For this review, take the finished solid that the model builds, in its own axes (mm). Face numbers are marked on the shaded views. A direction names the side the tool comes from. Round coordinates to 2 decimals unless told otherwise and drop trailing zeros. Order: outer loops, then holes, each group sorted by start corner. A loop starts at its lowest first (then second) coordinate and runs counter-clockwise, first axis right, second up. Notation, with made-up numbers: M 60,-21 L 92,-21 A22 ccw 92,3 Z; hole C -24,-18 d4. An arc over 180 degrees is marked long. Answer as a JSON object with one key per item and string values.
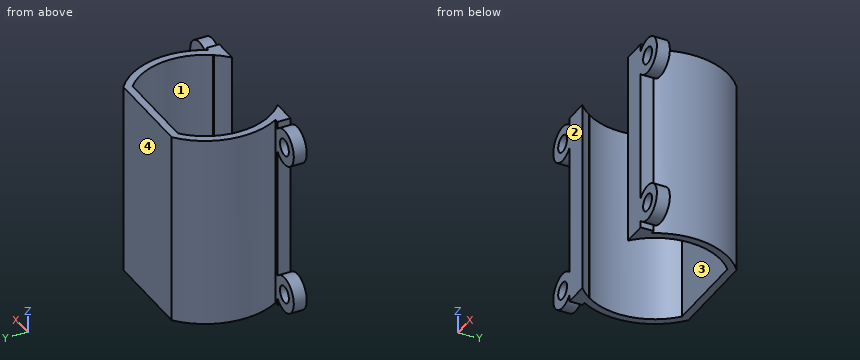
from build123d import *

# Parameters (mm, degrees)
SALIENTE_EXTRUIR1_DEPTH   = 30
VACIADO1_T                = 1.2
CROQUIS2_W                = 41.64599518
CROQUIS2_H                = 31.401201606
CORTAR_EXTRUIR1_DEPTH     = 1.3
CROQUIS3_W                = 19.002401527
CROQUIS3_H                = 2.972205444
CORTAR_EXTRUIR2_DEPTH     = 48.3
CROQUIS4_R                = 2.75
CROQUIS4_R_2              = 1.3
SALIENTE_EXTRUIR2_DEPTH   = 2
SALIENTE_EXTRUIR2_2_DEPTH = 2
SALIENTE_EXTRUIR2_3_DEPTH = 2
SALIENTE_EXTRUIR2_4_DEPTH = 2
CROQUIS5_W                = 2.061100057
CROQUIS5_H                = 29.9
SALIENTE_EXTRUIR3_DEPTH   = 2


with BuildPart() as part:
    # Croquis1 → Saliente-Extruir1 (new body)
    with BuildSketch(Plane.XY):
        with BuildLine():
            Line((-6.68954408, 7.7), (6.68954408, 7.7))
            ThreePointArc((6.68954408, 7.7), (10.2, 0), (6.68954408, -7.7))
            Line((6.68954408, -7.7), (-6.68954408, -7.7))
            ThreePointArc((-6.68954408, -7.7), (-10.2, 0), (-6.68954408, 7.7))
        make_face()
    extrude(amount=SALIENTE_EXTRUIR1_DEPTH)

    # Vaciado1
    vaciado1_openings = [part.faces().sort_by_distance(p)[0] for p in [
        (0, 0, 30),
    ]]
    offset(amount=VACIADO1_T, openings=vaciado1_openings, kind=Kind.INTERSECTION)

    # Croquis2 → Cortar-Extruir1 (cut)
    with BuildSketch(Plane(origin=(0, 0, -1.2), x_dir=(-1, 0, 0), z_dir=(0, 0, -1))):
        Rectangle(CROQUIS2_W, CROQUIS2_H)
    extrude(amount=-CORTAR_EXTRUIR1_DEPTH, mode=Mode.SUBTRACT)

    # Croquis3 → Cortar-Extruir2 (cut)
    with BuildSketch(Plane.XY.offset(30)):
        with Locations((-0.191367802, -9.186102722)):
            Rectangle(CROQUIS3_W, CROQUIS3_H)
    extrude(amount=-CORTAR_EXTRUIR2_DEPTH, mode=Mode.SUBTRACT)



with BuildPart() as body_2:
    # Croquis4 → Saliente-Extruir2 (new body)
    with BuildSketch(Plane.XZ.offset(7.7)):
        with Locations(Location((12.5, 3, 0), (0, 0, 270))):
            Circle(CROQUIS4_R)
        with Locations(Location((12.5, 3, 0), (0, 0, 270))):
            Circle(CROQUIS4_R_2, mode=Mode.SUBTRACT)
    extrude(amount=-SALIENTE_EXTRUIR2_DEPTH)


with BuildPart() as body_3:
    # Croquis4 → Saliente-Extruir2 2 (new body)
    with BuildSketch(Plane.XZ.offset(7.7)):
        with Locations(Location((12.5, 27, 0), (0, 0, 90))):
            Circle(CROQUIS4_R)
        with Locations(Location((12.5, 27, 0), (0, 0, 90))):
            Circle(CROQUIS4_R_2, mode=Mode.SUBTRACT)
    extrude(amount=-SALIENTE_EXTRUIR2_2_DEPTH)


with BuildPart() as body_4:
    # Croquis4 → Saliente-Extruir2 3 (new body)
    with BuildSketch(Plane.XZ.offset(7.7)):
        with Locations(Location((-12.5, 27, 0), (0, 0, 270))):
            Circle(CROQUIS4_R)
        with Locations(Location((-12.5, 27, 0), (0, 0, 270))):
            Circle(CROQUIS4_R_2, mode=Mode.SUBTRACT)
    extrude(amount=-SALIENTE_EXTRUIR2_3_DEPTH)


with BuildPart() as body_5:
    # Croquis4 → Saliente-Extruir2 4 (new body)
    with BuildSketch(Plane.XZ.offset(7.7)):
        with Locations(Location((-12.5, 3, 0), (0, 0, 90))):
            Circle(CROQUIS4_R)
        with Locations(Location((-12.5, 3, 0), (0, 0, 90))):
            Circle(CROQUIS4_R_2, mode=Mode.SUBTRACT)
    extrude(amount=-SALIENTE_EXTRUIR2_4_DEPTH)


with BuildPart() as part_1:
    add(part.part)

    add(body_2.part)  # Saliente-Extruir3 merges body 2

    add(body_3.part)  # Saliente-Extruir3 merges body 3

    add(body_4.part)  # Saliente-Extruir3 merges body 4

    add(body_5.part)  # Saliente-Extruir3 merges body 5
    # Croquis5 → Saliente-Extruir3 (add)
    with BuildSketch(Plane.XZ.offset(7.7)):
        with Locations((-9.437095098, 15.05)):
            Rectangle(CROQUIS5_W, CROQUIS5_H)
        with Locations((9.437095098, 15.05)):
            Rectangle(CROQUIS5_W, CROQUIS5_H)
    extrude(amount=-SALIENTE_EXTRUIR3_DEPTH)


solid = part_1.part
1) Add section D-D on y = -4.5. State the section outline as (x, z) points.
Geometry check:
{"outline": "M -10.47,0.1 L -9.15,0.1 L -9.15,30 L -10.47,30 Z; M 9.15,0.1 L 10.47,0.1 L 10.47,30 L 9.15,30 Z"}
2) Add section C-C on z = 6.5. State the section outline as (x, y) points, and give its area (3 significant figures).
Geometry check:
{"outline": "M -10.47,-7.7 L -6.69,-7.7 A10.2 cw -8.41,-5.78 L -8.41,-5.7 L -8.46,-5.7 A10.2 cw -6.69,7.7 L 6.69,7.7 A10.2 cw 8.46,-5.7 L 8.41,-5.7 L 8.41,-5.78 A10.2 cw 6.69,-7.7 L 10.47,-7.7 L 10.47,-5.7 L 9.87,-5.7 A11.4 ccw 7.12,8.9 L -7.12,8.9 A11.4 ccw -9.87,-5.7 L -10.47,-5.7 Z", "area": "65.0 mm²"}
3) Add section A-A on x = 12.5. State the section outline as (y, z) points, and give its area (3 significant figures).
Geometry check:
{"outline": "M -7.7,0.25 L -5.7,0.25 L -5.7,1.7 L -7.7,1.7 Z; M -7.7,4.3 L -5.7,4.3 L -5.7,5.75 L -7.7,5.75 Z; M -7.7,24.25 L -5.7,24.25 L -5.7,25.7 L -7.7,25.7 Z; M -7.7,28.3 L -5.7,28.3 L -5.7,29.75 L -7.7,29.75 Z", "area": "11.6 mm²"}
4) Mouldability with a two-part tool opening along X and no side actions: class the marked faces 3 and 4 as +X half, -X half, draft (parallel to the pull), parting line (faces both ways), or undercut.
Geometry check:
{"face 3": "undercut", "face 4": "draft"}
5) Add section B-B on z = 27. State the section outline as (x, y) points, and give its area (3 significant figures).
Geometry check:
{"outline": "M -15.25,-7.7 L -13.8,-7.7 L -13.8,-5.7 L -15.25,-5.7 Z; M -11.2,-7.7 L -6.69,-7.7 A10.2 cw -8.41,-5.78 L -8.41,-5.7 L -8.46,-5.7 A10.2 cw -6.69,7.7 L 6.69,7.7 A10.2 cw 8.46,-5.7 L 8.41,-5.7 L 8.41,-5.78 A10.2 cw 6.69,-7.7 L 11.2,-7.7 L 11.2,-5.7 L 9.87,-5.7 A11.4 ccw 7.12,8.9 L -7.12,8.9 A11.4 ccw -9.87,-5.7 L -11.2,-5.7 Z; M 13.8,-7.7 L 15.25,-7.7 L 15.25,-5.7 L 13.8,-5.7 Z", "area": "73.7 mm²"}
6) Insertion check: P1, Ø0.9, axis at y = -6.5, z = 29.5, coming from the -X side; P2, Ø6, axis at x = 13.5, z = 16.5, coming from the +Y side; P3, Ø2, axis at x = 12.5, z = 3, coming from the -Y side; P4, Ø1.5, axis at x = -5, z = 19.5, coming from the -Y side. Each pin has a flat end and moves straight along its axis. Give the tip position at first contact, or say it passes through.
Geometry check:
{"P1": "stops at x = -14.33", "P2": "stops at y = 4.44", "P3": "passes through", "P4": "stops at y = 7.7"}
7) For L1, parallel to X at y = -7.3, z = 3; L2, parallel to X at y = -6.2, z = 3; L3, parallel to Y at x = -5, z = 13.5, list the stretches that pass through material, from the lowest coordinate up.
Geometry check:
{"L1": "x = -15.25 to -13.8, -11.2 to -7.12, 7.12 to 11.2, 13.8 to 15.25", "L2": "x = -15.25 to -13.8, -11.2 to -8.1, 8.1 to 11.2, 13.8 to 15.25", "L3": "y = 7.7 to 8.9"}
8) Machinability: for the marked faces 1 and 2, which of the approach directions +Z, -Z, +X, -X, +Y, -Y give a long, thin tool a straight path to every point of the face, cutting with its end or side? Answer none if there is none.
Geometry check:
{"face 1": "+Z, -Z", "face 2": "+Z, -Z, +X, -X, -Y"}
